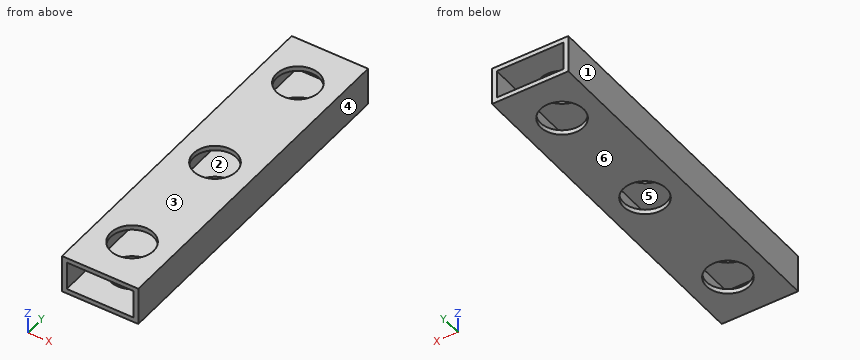
Autodesk Inventor part; units mm, degrees
ref_plane "YZ Plane" through (0, 0, 0) normal (1, 0, 0) x (0, 1, 0)
ref_plane "XZ Plane" through (0, 0, 0) normal (0, 1, 0) x (-1, 0, 0)
ref_plane "XY Plane" through (0, 0, 0) normal (0, 0, 1) x (1, 0, 0)
sketch "Sketch2" plane through (0, 0, 0) normal (0, 1, 0) x (-1, 0, 0)
  line L0 (0, 0) -> (50.8, 0)
  line L1 (50.8, 0) -> (50.8, -25.4)
  line L2 (50.8, -25.4) -> (0, -25.4)
  line L3 (0, -25.4) -> (0, 0)
  line L4 (47.625, -22.225) -> (47.625, -3.175)
  line L5 (47.625, -3.175) -> (3.175, -3.175)
  line L6 (3.175, -3.175) -> (3.175, -22.225)
  line L7 (3.175, -22.225) -> (47.625, -22.225)
  dimension "d4" = 50.8
  dimension "d5" = 25.4
  dimension "d6" = 3.175
extrude "Extrusion2" add sketch "Sketch2" along normal blind 228.6
sketch "Sketch3" plane through (-50.8, 0, 0) normal (0, 0, 1) x (1, 0, 0)
  circle A0 centre (25.4, 31.75) radius 14.2875
  line L0 (50.8, 0) -> (0, 0)
  line L1 (0, 0) -> (0, 228.6)
  circle A1 centre (25.4, 196.85) radius 14.2875
  line L2 (0, 228.6) -> (50.8, 228.6)
  circle A2 centre (25.4, 114.3) radius 14.2875
  dimension "d9" = 31.75
  dimension "d10" = 25.4
  dimension "d11" = 25.4
  dimension "d12" = 31.75
  dimension "d13" = 114.3
  dimension "d14" = 25.4
  dimension "d15" = 28.575
  dimension "d16" = 28.575
  dimension "d17" = 28.575
extrude "Extrusion3" cut sketch "Sketch3" against normal blind 50.8
properties part number "AluminumBar-1111-2020"
Model file for the job. Use its own axes, mm. Face numbers are marked on the shaded views. A direction names the side the tool comes from. Give positions to 0.01 mm unless a question says otherwise; leave off trailing zeros. Order: outer loops, then holes, each group sorted by start corner. A loop starts at its lowest first (then second) coordinate and runs counter-clockwise, first axis right, second up. Notation, with made-up numbers: M 72.5,23.25 L 77.5,23.25 A26 cw 77.5,49.25 Z; hole C 56.5,8.5 d8. An arc over 180 degrees is marked long. Write item = value, one per line.
Q1. Cut at D-D, the plane z = -9.5. List the corners of the cut face in (x, y) (3 decimals), then the cut area to 3 significant figures.
Derived:
outline = M -50.8,0 L -47.625,0 L -47.625,228.6 L -50.8,228.6 Z; M -3.175,0 L 0,0 L 0,228.6 L -3.175,228.6 Z
area = 1,450 mm2
Q2. Cut at C-C, the plane x = -25.4. Count the separate pieces of the cut face and the enclosed holes in it, then the cut area to 3 significant figures.
Derived:
separate_pieces = 8
enclosed_holes = 0
area = 907 mm2
Q3. Cut at B-B, the plane y = 114.3. List the corners of the cut face in (x, z) (1 decimal), then the cut area to 3 significant figures.
Derived:
outline = M -50.8,-25.4 L -39.7,-25.4 L -39.7,-22.2 L -47.6,-22.2 L -47.6,-3.2 L -39.7,-3.2 L -39.7,0 L -50.8,0 Z; M -11.1,-25.4 L 0,-25.4 L 0,0 L -11.1,0 L -11.1,-3.2 L -3.2,-3.2 L -3.2,-22.2 L -11.1,-22.2 Z
area = 262 mm2
Q4. Cut at A-A, the plane x = -6.5. List the corners of the cut face in (y, z) (3 decimals), then the cut area to 3 significant figures.
Derived:
outline = M 0,-25.4 L 228.6,-25.4 L 228.6,-22.225 L 0,-22.225 Z; M 0,-3.175 L 228.6,-3.175 L 228.6,0 L 0,0 Z
area = 1,450 mm2
Q5. Flat gauge pin, fed straight in: pin 1 (1.5 mm diameter, centred on x = -41.5, z = -22, fed in from -Y). Where does the tip first touch, or does it go through?
Derived:
pin_1 = 0
Q6. Two-plate mould, pull along Z, no slides. Class the marked faces 3, 4, 5 and 6: pulls with the +Z half, pulls with the -Z half, needs draft (parallel to the pull), parting line crosses it, or undercut.
Derived:
face_3 = pulls with the +Z half
face_4 = needs draft
face_5 = undercut
face_6 = pulls with the -Z half
Q7. Drill centre lines: line 1 (Y direction, x = -25.4, z = -2.2); line 2 (X direction, y = 58, z = -7.5) (3 decimals); line 3 (Z direction, x = -31, y = 57) (3 decimals). Where is each one in solid material? Low to high. Write a range as [from, to].
Derived:
line_1 = [0, 17.46], [46.04, 100.01], [128.59, 182.56], [211.14, 228.6]
line_2 = [-50.8, -47.625], [-3.175, 0]
line_3 = [-25.4, -22.225], [-3.175, 0]
Q8. Tool access for the marked faces 1 and 2: list every direction of +Z, -Z, +X, -X, +Y, -Y with a clear straight run to the whole face (end or side of a thin tool).
Derived:
face_1 = +Z, -Z, -X, +Y, -Y
face_2 = +Y, -Y
